```python
from build123d import *

# Parameters (mm, degrees)
F1_DEPTH = 15
F2_R     = 5
F3_R     = 5
F4_SIZE  = 5


with BuildPart() as f1:
    # F0 (on Front) → F1 (new body)
    with BuildSketch(Plane.XZ):
        Polygon((285, 0), (0, 0), (-285, 0), (-285, -17.5), (-300, -17.5), (-300, -32.5), (-285, -32.5), (-285, -50), (0, -50), (285, -50), (285, -32.5), (300, -32.5), (300, -17.5), (285, -17.5), align=None)
    extrude(amount=F1_DEPTH)

    # F2
    f2_edges = [f1.edges().sort_by_distance(p)[0] for p in [
        (300, 0, -25),
        (-300, 0, -25),
    ]]
    fillet(f2_edges, radius=F2_R)

    # F3
    f3_edges = [f1.edges().sort_by_distance(p)[0] for p in [
        (0, 0, 0),
        (0, 0, -50),
    ]]
    fillet(f3_edges, radius=F3_R)

    # F4
    f4_edges = [f1.edges().sort_by_distance(p)[0] for p in [
        (0, -15, -50),
    ]]
    chamfer(f4_edges, length=F4_SIZE)


solid = f1.part
```
The model under review builds one solid part; all positions refer to its coordinate system, in mm. A direction names the side the tool comes from. Round coordinates to 2 decimals unless told otherwise and drop trailing zeros. Loops run counter-clockwise (first coordinate to the right, second up) from the corner with the lowest first, then second, coordinate; pieces in that order, holes last. Notation, with made-up numbers: (-21, -34.5) -> (35, -34.5) arc R18 cw to (35, -14.5) -> close; hole circle Ø9 at (-7.75, 4). An arc over 180 degrees is marked (long way). Answer in a Markdown table with one row per item.
1) Wall thickness on line 1 along X through (y, z) = (-0.75, -40); line 2 along X through (y, z) = (-4, -20.5); line 3 along Z through (x, y) = (-209, -3.25): over which ranges is each line inside the solid? List them lowest first.
Taken from the geometry:
| item | result |
|---|---|
| line 1 | x = -285 to 285 |
| line 2 | x = -299.9 to 299.9 |
| line 3 | z = -49.68 to -0.32 |
2) Tool access review of faces 1 (the flat face through (-285, -7, -9)), 2 (the flat face through (-293, -7, -32.5)), 3 (the flat face through (285, -7, -9)): name each direction out of +Z, -Z, +X, -X, +Y, -Y from which nothing blocks a thin tool from reaching the whole face with its end or side.
Taken from the geometry:
| item | result |
|---|---|
| face 1 | +Z, -X, +Y, -Y |
| face 2 | -Z, -X, +Y, -Y |
| face 3 | +Z, +X, +Y, -Y |
3) Consider section B-B, the plane x = -115.5. Write out the cut boundary in (y, z), plus the area to 3 significant figures.
Taken from the geometry:
| item | result |
|---|---|
| outline | (-15, -45) -> (-10, -50) -> (-5, -50) arc R5 ccw to (0, -45) -> (0, -5) arc R5 ccw to (-5, 0) -> (-15, 0) -> close |
| area | 727 mm² |
4) Consider section A-A, the plane y = -12.25. Write out the cut boundary in (x, z), plus the area to 3 significant figures.
Taken from the geometry:
| item | result |
|---|---|
| outline | (-300, -32.5) -> (-285, -32.5) -> (-285, -47.75) -> (285, -47.75) -> (285, -32.5) -> (300, -32.5) -> (300, -17.5) -> (285, -17.5) -> (285, 0) -> (-285, 0) -> (-285, -17.5) -> (-300, -17.5) -> close |
| area | 27,700 mm² |
5) For pin 1 Ø4.5 at (x, y) = (292.5, -4.5) entering from +Z; pin 2 Ø4.5 at (x, y) = (-293.5, -8) entering from -Z, all flat-tipped, find the tip position at first contact; note any pin that passes through.
Taken from the geometry:
| item | result |
|---|---|
| pin 1 | stops at z = -17.5 |
| pin 2 | stops at z = -32.5 |
